```python
from build123d import *

# Parameters (mm, degrees)
EXTRUDE_START       = -21
EXTRUDE_1_DEPTH     = 10.25
EXTRUDE_START_2     = -51.75
EXTRUDE_2_DEPTH     = 10.25
EXTRUDE_START_3     = -31.25
EXTRUDE_3_DEPTH     = 20.5
CUT_EXTRUDE_START   = -21
SKETCH_7_R          = 1.275
CUT_EXTRUDE_4_DEPTH = 5
FILLET_1_R          = 0.5
FILLET_2_R          = 0.5


with BuildPart() as part:
    # Sketch 3 → Revolve 1 (revolve)
    with BuildSketch(Plane(origin=(0, 0, 0), x_dir=(0, 0, -1), z_dir=(1, 0, 0)), mode=Mode.PRIVATE) as revolve_1_sk:
        Polygon((0, 2), (0, 0), (21, 0), (21, 2.5), (0.5, 2.5), align=None)
        Polygon((19, 4.5), (21, 4.5), (21, 11), (19.5, 11), (19, 10.5), align=None)
    revolve(revolve_1_sk.sketch.rotate(Axis((0, 0, -21), (0, 0, 1)), 90), axis=Axis((0, 0, -21), (0, 0, 1)))

    # Sketch 4 → Extrude 1 (add)
    with BuildSketch(Plane.XY.offset(EXTRUDE_START)):
        with BuildLine():
            Line((16.970562748, 21), (-16.970562748, 21))
            ThreePointArc((-16.970562748, 21), (-19.091883092, 19.091883092), (-21, 16.970562748))
            Line((-21, 16.970562748), (-21, -16.970562748))
            ThreePointArc((-21, -16.970562748), (-19.091883092, -19.091883092), (-16.970562748, -21))
            Line((-16.970562748, -21), (16.970562748, -21))
            ThreePointArc((16.970562748, -21), (19.091883092, -19.091883092), (21, -16.970562748))
            Line((21, -16.970562748), (21, 16.970562748))
            ThreePointArc((21, 16.970562748), (19.091883092, 19.091883092), (16.970562748, 21))
        make_face()
    extrude(amount=-EXTRUDE_1_DEPTH)



with BuildPart() as body_2:
    # Sketch 4_2 → Extrude 2 (new body)
    with BuildSketch(Plane.XY.offset(EXTRUDE_START_2)):
        with BuildLine():
            Line((16.970562748, 21), (-16.970562748, 21))
            ThreePointArc((-16.970562748, 21), (-19.091883092, 19.091883092), (-21, 16.970562748))
            Line((-21, 16.970562748), (-21, -16.970562748))
            ThreePointArc((-21, -16.970562748), (-19.091883092, -19.091883092), (-16.970562748, -21))
            Line((-16.970562748, -21), (16.970562748, -21))
            ThreePointArc((16.970562748, -21), (19.091883092, -19.091883092), (21, -16.970562748))
            Line((21, -16.970562748), (21, 16.970562748))
            ThreePointArc((21, 16.970562748), (19.091883092, 19.091883092), (16.970562748, 21))
        make_face()
    extrude(amount=-EXTRUDE_2_DEPTH)


with BuildPart() as part_1:
    add(part.part)

    add(body_2.part)  # Extrude 3 merges body 2
    # Sketch 5 → Extrude 3 (add)
    with BuildSketch(Plane.XY.offset(EXTRUDE_START_3)):
        with BuildLine():
            Line((20, -12.338962679), (20, 12.338962679))
            ThreePointArc((20, 12.338962679), (16.617009358, 16.617009358), (12.338962679, 20))
            Line((12.338962679, 20), (-12.338962679, 20))
            ThreePointArc((-12.338962679, 20), (-16.617009358, 16.617009358), (-20, 12.338962679))
            Line((-20, 12.338962679), (-20, -12.338962679))
            ThreePointArc((-20, -12.338962679), (-16.617009358, -16.617009358), (-12.338962679, -20))
            Line((-12.338962679, -20), (12.338962679, -20))
            ThreePointArc((12.338962679, -20), (16.617009358, -16.617009358), (20, -12.338962679))
        make_face()
    extrude(amount=-EXTRUDE_3_DEPTH)

    # Sketch 7 → Cut-Extrude 4 (cut)
    with BuildSketch(Plane.XY.offset(CUT_EXTRUDE_START)):
        with Locations((-15.5, 15.5)):
            Circle(SKETCH_7_R)
        with Locations((15.5, 15.5)):
            Circle(SKETCH_7_R)
        with Locations((15.5, -15.5)):
            Circle(SKETCH_7_R)
        with Locations((-15.5, -15.5)):
            Circle(SKETCH_7_R)
    extrude(amount=-CUT_EXTRUDE_4_DEPTH, mode=Mode.SUBTRACT)

    # Fillet 1
    fillet_1_edges = [part_1.edges().sort_by_distance(p)[0] for p in [
        (19.091883092, 19.091883092, -21),
        (0, 21, -21),
        (-19.091883092, 19.091883092, -21),
        (-21, 0, -21),
        (-19.091883092, -19.091883092, -21),
        (0, -21, -21),
        (19.091883092, -19.091883092, -21),
        (21, 0, -21),
        (19.091883092, 19.091883092, -31.25),
        (16.970562748, 21, -26.125),
        (21, 0, -31.25),
        (21, 16.970562748, -26.125),
        (19.091883092, -19.091883092, -31.25),
        (21, -16.970562748, -26.125),
        (0, -21, -31.25),
        (16.970562748, -21, -26.125),
        (-19.091883092, -19.091883092, -31.25),
        (-16.970562748, -21, -26.125),
        (-21, 0, -31.25),
        (-21, -16.970562748, -26.125),
        (-19.091883092, 19.091883092, -31.25),
        (-21, 16.970562748, -26.125),
        (0, 21, -31.25),
        (-16.970562748, 21, -26.125),
    ]]
    fillet(fillet_1_edges, radius=FILLET_1_R)

    # Fillet 2
    fillet_2_edges = [part_1.edges().sort_by_distance(p)[0] for p in [
        (19.091883092, 19.091883092, -62),
        (16.970562748, 21, -56.875),
        (21, 0, -62),
        (21, 16.970562748, -56.875),
        (19.091883092, -19.091883092, -62),
        (21, -16.970562748, -56.875),
        (0, -21, -62),
        (16.970562748, -21, -56.875),
        (-19.091883092, -19.091883092, -62),
        (-16.970562748, -21, -56.875),
        (-21, 0, -62),
        (-21, -16.970562748, -56.875),
        (-19.091883092, 19.091883092, -62),
        (-21, 16.970562748, -56.875),
        (0, 21, -62),
        (-16.970562748, 21, -56.875),
        (19.091883092, 19.091883092, -51.75),
        (0, 21, -51.75),
        (-19.091883092, 19.091883092, -51.75),
        (-21, 0, -51.75),
        (-19.091883092, -19.091883092, -51.75),
        (0, -21, -51.75),
        (19.091883092, -19.091883092, -51.75),
        (21, 0, -51.75),
    ]]
    fillet(fillet_2_edges, radius=FILLET_2_R)


solid = part_1.part
```
Verification items for the finished model (mm, model axes). A direction names the side the tool comes from. Coordinates: 2 decimals unless noted, no trailing zeros. Write each loop counter-clockwise with the first axis right and the second up, starting at its lowest first coordinate (ties: lowest second). Pieces come first, ordered by that corner, then holes. Notation, with made-up numbers: M -3.5,77 L 22.5,77 A30 ccw 22.5,116 Z; hole C 79,9.25 d4. An arc over 180 degrees is marked long. Answer as a JSON object with one key per item and string values. Group by question number.
(1) Cross-section at B-B, the plane z = -47.5. Record the cut outline in (x, y).
(2) Tool access check on faces 4 (the face through (2.38, 10.74, -20.24)), 5 (the face through (-17, 17, -31.25)), 6 (the face through (-16.671, -16.563, -41.356)), 7 (the face through (-20, 0, -41)). Record the directions out of +Z, -Z, +X, -X, +Y, -Y that give a thin tool (end or side, any length) a straight path to the whole face; none if there is none.
(3) Material ranges on line 1 (Y direction, x = 0, z = -20.5); line 2 (Y direction, x = -15.5, z = -22.55) (3 decimals); line 3 (X direction, y = 15, z = -23), recorded low to high.
(4) Gauge pin test, flat ends, axial feed: pin 1 (3 mm diameter, centred on x = 16, y = -15, fed in from +Z); pin 2 (8 mm diameter, centred on x = 2.5, z = -37.5, fed in from +Y); pin 3 (1.3 mm diameter, centred on x = -16, y = -15.5, fed in from +Z). Record the tip position at first contact, or that the pin passes through.
(5) Cross-section at A-A, the plane y = -15.5. Record the cut outline in (x, z) (3 decimals).
(6) Release check for a two-part mould opening along Z. For faces 1 (the face through (0, 0, -62)), 2 (the face through (-17, 17, -51.75)), 3 (the face through (14.56, -14.64, -23.46)) record: +Z half, -Z half, draft (parallel to the pull), parting line (faces both ways), or undercut.
Reply:
{
 "1": {"outline": "M -20,-12.34 A23.5 ccw -12.34,-20 L 12.34,-20 A23.5 ccw 20,-12.34 L 20,12.34 A23.5 ccw 12.34,20 L -12.34,20 A23.5 ccw -20,12.34 Z"},
 "2": {"face 4": "+Z", "face 5": "none", "face 6": "-X, -Y", "face 7": "-X, +Y, -Y"},
 "3": {"line 1": "-11 to -4.5, -2.5 to 2.5, 4.5 to 11", "line 2": "-21 to -16.775, -14.225 to 14.225, 16.775 to 21", "line 3": "-21 to -16.67, -14.33 to 14.33, 16.67 to 21"},
 "4": {"pin 1": "z = -21", "pin 2": "y = 20", "pin 3": "z = -26"},
 "5": {"outline": "M -21,-61.5 A0.5 ccw -20.5,-62 L 20.5,-62 A0.5 ccw 21,-61.5 L 21,-52.25 A0.5 ccw 20.5,-51.75 L 17.664,-51.75 L 17.664,-31.25 L 20.5,-31.25 A0.5 ccw 21,-30.75 L 21,-21.5 A0.5 ccw 20.5,-21 L 16.775,-21 L 16.775,-26 L 14.225,-26 L 14.225,-21 L -14.225,-21 L -14.225,-26 L -16.775,-26 L -16.775,-21 L -20.5,-21 A0.5 ccw -21,-21.5 L -21,-30.75 A0.5 ccw -20.5,-31.25 L -17.664,-31.25 L -17.664,-51.75 L -20.5,-51.75 A0.5 ccw -21,-52.25 Z"},
 "6": {"face 1": "-Z half", "face 2": "undercut", "face 3": "draft"}
}
